Source: CAD feature listing. Evaluate the final solid. Frame: model axes, mm. A direction names the side the tool comes from. Coordinates: 2 decimals unless noted, no trailing zeros. Order: outer loops, then holes, each group sorted by start corner. A loop starts at its lowest first (then second) coordinate and runs counter-clockwise, first axis right, second up. Notation, with made-up numbers: (84, 72) -> (101, 72) arc R22 cw to (101, 98) -> close; hole circle Ø6 at (44, -37). An arc over 180 degrees is marked (long way). Write item = value, one per line. Start each with the question number.
Item 1: Mould query, pull axis Y, two halves, no side actions, for faces 1 (the cylindrical face through (-11.34, 65.89, 0.5)), 2 (the flat face through (54, -28, 0)), 3 (the flat face through (0, 58.1, -11.4)). Classes: released by +Y, released by -Y, zero draft, split by the parting line, or undercut.
Item 2: Section query B-B (x = -20). Output: boundary loops of the cut face in (y, z).
Item 3: Section query A-A (z = 0). Output: boundary loops of the cut face in (x, y), then the cut area to 3 significant figures.
Item 4: Set-up query: faces 4 (the flat face through (43, 0, 4)), 5 (the flat face through (-28, 55, 0)). Return all of +Z, -Z, +X, -X, +Y, -Y with unobstructed straight access to the full face (end or side cutting, diameter ignored); none if empty.
Item 5: Ray query, line 1 along X through (y, z) = (-12, 10); line 2 along Y through (x, z) = (61.5, 6); line 3 along Y through (x, z) = (42.5, -3). Return the intervals inside material, ascending. Write a range as [from, to].
Item 6: Contact query for flat-ended pins moving along their axis: pin 1 (10 mm diameter, centred on x = -14.5, z = 9, fed in from +Y); pin 2 (5 mm diameter, centred on x = 29, z = 7, fed in from -Y); pin 3 (4 mm diameter, centred on y = 24, z = 9.5, fed in from +X); pin 4 (5 mm diameter, centred on x = 16, y = 29.5, fed in from -Z). Output: stop coordinate, or through.
```python
from build123d import *

# Parameters (mm, degrees)
F1_R     = 17.5
F3_R     = 11.4
F4_DEPTH = 28
F5_R     = 11.4
F6_DEPTH = 28
F7_R     = 5
F8_R     = 5


with BuildPart() as f2:
    # F2: sweep along a path in F0
    with BuildLine(Plane.XY) as f2_path:
        ThreePointArc((0, 54.5), (38.5373195747, 38.5373195747), (54.5, 0))
    # F1 (on Right) → F2 (sweep)
    with BuildSketch(Plane.YZ):
        with Locations((54.5, 0)):
            Circle(F1_R)
    sweep(path=f2_path.line)

    # F3 (on face) → F4 (join)
    with BuildSketch(Plane.XZ):
        with Locations((54.5, 0)):
            Circle(F3_R)
    extrude(amount=F4_DEPTH)

    # F5 (on face) → F6 (join)
    with BuildSketch(Plane(origin=(0, 0, 0), x_dir=(0, -1, 0), z_dir=(-1, 0, 0))):
        with Locations((-54.5, 0)):
            Circle(F5_R)
    extrude(amount=F6_DEPTH)

    # F7
    f7_edges = [f2.edges().sort_by_distance(p)[0] for p in [
        (43.1, -28, 0),
    ]]
    fillet(f7_edges, radius=F7_R)

    # F8
    f8_edges = [f2.edges().sort_by_distance(p)[0] for p in [
        (-28, 65.9, 0),
    ]]
    fillet(f8_edges, radius=F8_R)


solid = f2.part
```
Computed:
q1.face_1 = split by the parting line
q1.face_2 = released by -Y
q1.face_3 = zero draft
q2.outline = circle Ø22.8 at (54.5, 0)
q3.outline = (-28, 48.1) arc R5 ccw to (-23, 43.1) -> (0, 43.1) -> (0, 37) arc R37 cw to (37, 0) -> (43.1, 0) -> (43.1, -23) arc R5 ccw to (48.1, -28) -> (60.9, -28) arc R5 ccw to (65.9, -23) -> (65.9, 0) -> (72, 0) arc R72 ccw to (0, 72) -> (0, 65.9) -> (-23, 65.9) arc R5 ccw to (-28, 60.9) -> close
q3.area = 4,250 mm^2
q4.face_4 = -Y
q4.face_5 = +Z, -Z, -X, +Y, -Y
q5.line_1 = [49.03, 59.97]
q5.line_2 = [-27.13, 35.36]
q5.line_3 = [0, 57.8]
q6.pin_1 = 65.18
q6.pin_2 = 21.67
q6.pin_3 = 66.31
q6.pin_4 = through
